For this review, use the dimensioned drawing (mm, ordinates from the lowest corner) and the shaded views. A direction names the side the tool comes from. Coordinates: 2 decimals unless noted, no trailing zeros. Write each loop counter-clockwise with the first axis right and the second up, starting at its lowest first coordinate (ties: lowest second). Pieces come first, ordered by that corner, then holes. Notation, with made-up numbers: (46.5, 44) - (71.5, 44) arc R31 ccw to (71.5, 70) - close; hole circle Ø4 at (64.25, 58.5). An arc over 180 degrees is marked (long way). Use one line per item in the form item = value. Start each with the question number.
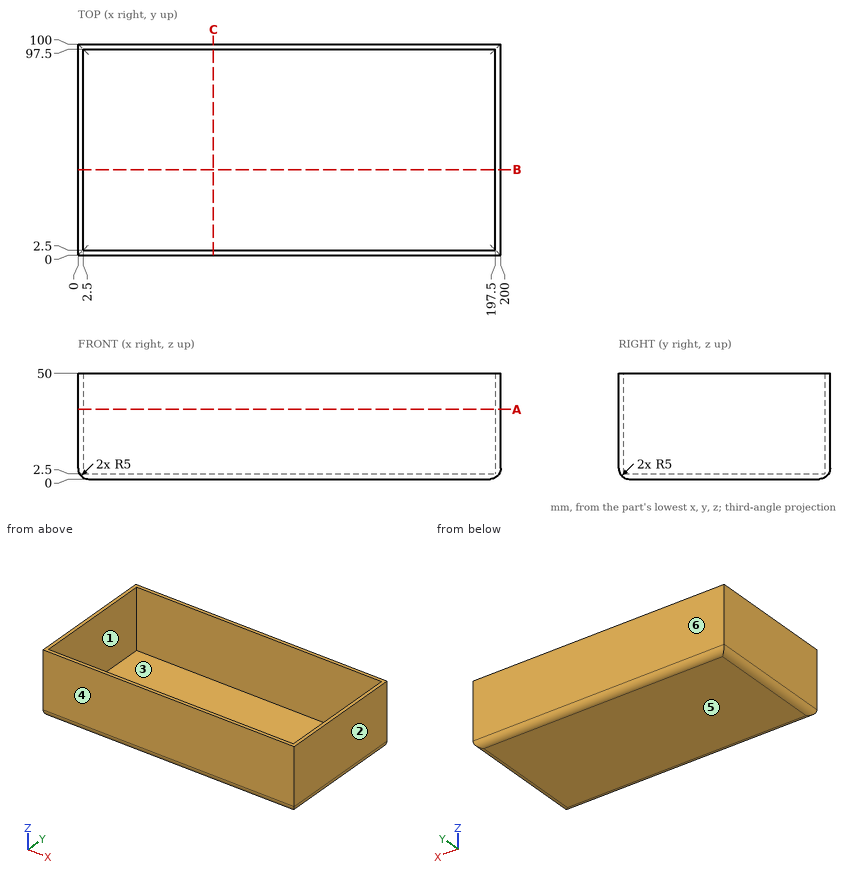
1. For L1, parallel to Y at x = 89, z = 28.5; L2, parallel to X at y = 13.5, z = 38.5; L3, parallel to Z at x = 29.5, y = 61, list the stretches that pass through material, from the lowest coordinate up.
2. For the marked faces 1 and 2, list the 3-axis set-ups (+Z, -Z, +X, -X, +Y, -Y) from which the entire face can be reached by the end or side of a thin tool; tool diameter is ignored.
3. Take a section at C-C (x = 64). State the section outline as (y, z) points.
4. Take a section at A-A (z = 33). State the section outline as (x, y) points.
5. For P1, Ø12, axis at x = 123, y = 45.5, coming from the -Z side; P2, Ø12, axis at x = 102, y = 21, coming from the +Z side, all flat-tipped, find the tip position at first contact; note any pin that passes through.
6. The part is to be moulded in two halves that separate along Y. For the marked faces 3, 4, 5 and 6, say which applies: released by +Y, released by -Y, zero draft, split by the parting line, or undercut.
7. Take a section at B-B (y = 40.5). State the section outline as (x, z) points, plus the area to 3 significant figures.
Returned:
q1.L1 = 0 to 2.5, 97.5 to 100
q1.L2 = 0 to 2.5, 197.5 to 200
q1.L3 = 0 to 2.5
q2.face_1 = +Z
q2.face_2 = +Z, -Z, +X, +Y, -Y
q3.outline = (0, 5) arc R5 ccw to (5, 0) - (95, 0) arc R5 ccw to (100, 5) - (100, 50) - (97.5, 50) - (97.5, 2.5) - (2.5, 2.5) - (2.5, 50) - (0, 50) - close
q4.outline = (0, 0) - (200, 0) - (200, 100) - (0, 100) - close; hole (2.5, 2.5) - (197.5, 2.5) - (197.5, 97.5) - (2.5, 97.5) - close
q5.P1 = 0
q5.P2 = 2.5
q6.face_3 = undercut
q6.face_4 = released by -Y
q6.face_5 = zero draft
q6.face_6 = released by +Y
q7.outline = (0, 5) arc R5 ccw to (5, 0) - (195, 0) arc R5 ccw to (200, 5) - (200, 50) - (197.5, 50) - (197.5, 2.5) - (2.5, 2.5) - (2.5, 50) - (0, 50) - close
q7.area = 727 mm²
